Read the model definition and answer for the solid it produces. Units are mm, in the model's axes. A direction names the side the tool comes from. Round coordinates to 2 decimals unless told otherwise and drop trailing zeros. Write each loop counter-clockwise with the first axis right and the second up, starting at its lowest first coordinate (ties: lowest second). Pieces come first, ordered by that corner, then holes.
from build123d import *

# Parameters (mm, degrees)
F1_DEPTH = 65.0748
F3_DEPTH = 69.851
F4_R     = 17.4498
F5_DEPTH = 25.4
F6_R     = 6.35
F7_DEPTH = 30.1498
F8_R     = 3.175
F9_DEPTH = 15.875
F10_F1_R = 3.175
F10_F2_R = 3.175


with BuildPart() as f1:
    # F0 (on Right) → F1 (new body)
    with BuildSketch(Plane.YZ):
        Polygon((32.8030504316, 53.1119473694), (-37.0469495684, 53.1119473694), (-37.0469495684, 8.6619473694), (-14.8219495684, 8.6619473694), (-14.8219495684, -4.1650526306), (-9.2339495684, -4.1650526306), (-9.2339495684, -8.9275526306), (-14.8219495684, -8.9275526306), (-14.8219495684, -29.4380526306), (10.5780504316, -29.4380526306), (10.5780504316, -8.9275526306), (4.9900504316, -8.9275526306), (4.9900504316, -4.1650526306), (10.5780504316, -4.1650526306), (10.5780504316, 8.6619473694), (32.8030504316, 8.6619473694), align=None)
    extrude(amount=F1_DEPTH)

    # F2 (on face) → F3 (cut, through all)
    with BuildSketch(Plane.XZ.offset(37.0469495684)):
        with BuildLine():
            ThreePointArc((22.225, 5.4869473694), (24.4700640303, 6.4168833391), (25.4, 8.6619473694))
            Line((25.4, 8.6619473694), (0, 8.6619473694))
            Line((0, 8.6619473694), (0, -29.4380526306))
            Line((0, -29.4380526306), (9.525, 5.4869473694))
            Line((9.525, 5.4869473694), (22.225, 5.4869473694))
        make_face()
        Polygon((25.4, 27.7119473694), (25.4, 53.1119473694), (0, 53.1119473694), (0, 8.6619473694), (25.4, 8.6619473694), align=None)
        with BuildLine():
            Line((65.0748, 53.1119473694), (39.8529659904, 53.1119473694))
            ThreePointArc((39.8529659904, 53.1119473694), (51.2636522621, 42.3660722249), (56.8255061373, 27.7119473694))
            Line((56.8255061373, 27.7119473694), (65.0748, 27.7119473694))
            Line((65.0748, 27.7119473694), (65.0748, 53.1119473694))
        make_face()
    extrude(amount=-F3_DEPTH, mode=Mode.SUBTRACT)

    # F4 (on face) → F5 (join)
    with BuildSketch(Plane.YZ.offset(65.0748)):
        with Locations((-2.1219495684, 26.1117473694)):
            Circle(F4_R)
    extrude(amount=-F5_DEPTH)

    # F6 (on face) → F7 (cut)
    with BuildSketch(Plane.YZ.offset(65.0748)):
        with Locations((-2.1219495684, 26.1117473694)):
            Circle(F6_R)
    extrude(amount=-F7_DEPTH, mode=Mode.SUBTRACT)

    # F8 (on face) → F9 (cut)
    with BuildSketch(Plane(origin=(25.4, 0, 0), x_dir=(0, -1, 0), z_dir=(-1, 0, 0))):
        with Locations((-16.9280504316, 34.0619473694)):
            Circle(F8_R)
        with Locations((21.1719495684, 34.0619473694)):
            Circle(F8_R)
    extrude(amount=-F9_DEPTH, mode=Mode.SUBTRACT)

    # F10: fillet of radius 3.175 on 12 edges, made by hand

    # F10_f1
    f10_f1_edges = [f1.edges().sort_by_distance(p)[0] for p in [
        (50.428197841, -2.1264417395, 43.5615467912),
        (56.8255061373, -28.2725863076, 27.7119473694),
        (56.8255061373, 24.0286871709, 27.7119473694),
    ]]
    fillet(f10_f1_edges, radius=F10_F1_R)

    # F10_f2
    f10_f2_edges = [f1.edges().sort_by_distance(p)[0] for p in [
        (50.5351306509, -37.0469495684, 43.4143386342),
        (62.2832541328, -37.0469495684, 27.7119473694),
        (65.0748, 32.8030504316, 18.1869473694),
        (50.5351306509, 32.8030504316, 43.4143386342),
        (39.8529659904, -2.1219495684, 53.1119473694),
        (65.0748, -28.2725863076, 27.7119473694),
        (65.0748, -2.1219495684, 43.5615473694),
        (65.0748, 24.0286871709, 27.7119473694),
        (65.0748, -37.0469495684, 18.1869473694),
        (57.4937274099, 32.8030504316, 28.4194187475),
        (57.4937274099, -37.0469495684, 28.4194187475),
    ]]
    fillet(f10_f2_edges, radius=F10_F2_R)


solid = f1.part
Q1. Which of the six approach directions +Z, -Z, +X, -X, +Y, -Y give full straight-line access (tool end or side, diameter ignored) to faces 1 (the cylindrical face through (48.77, -2.57, 45.66)), 2 (the cylindrical face through (64.169, -26.919, 26.757)), 3 (the flat face through (45, 22, 8.662))?
Verdict:
face 1: +Z, +X
face 2: +Z, +X, -Y
face 3: -Z, +X, -X, +Y
Q2. Determine the mould class of faces 4 (the flat face through (16, -2, 5.487)), 5 (the flat face through (39, -37.047, 26)), 6 (the cylindrical face through (33.226, -22.637, 31.245)) for opening direction Z: pulls with the +Z half, pulls with the -Z half, needs draft (parallel to the pull), parting line crosses it, or undercut.
Verdict:
face 4: pulls with the +Z half
face 5: needs draft
face 6: undercut
Q3. Section A-A (x = 21) is taken. Determine the outline of the cut face in (y, z), then the cut area to 3 significant figures.
Verdict:
outline: (-14.82, -29.44) - (10.58, -29.44) - (10.58, -8.93) - (4.99, -8.93) - (4.99, -4.17) - (10.58, -4.17) - (10.58, 5.49) - (-14.82, 5.49) - (-14.82, -4.17) - (-9.23, -4.17) - (-9.23, -8.93) - (-14.82, -8.93) - close
area: 834 mm2
Q4. Section D-D (x = 8.5) is taken. Determine the outline of the cut face in (y, z), then the cut area to 3 significant figures.
Verdict:
outline: (-14.82, -29.44) - (10.58, -29.44) - (10.58, -8.93) - (4.99, -8.93) - (4.99, -4.17) - (10.58, -4.17) - (10.58, 1.73) - (-14.82, 1.73) - (-14.82, -4.17) - (-9.23, -4.17) - (-9.23, -8.93) - (-14.82, -8.93) - close
area: 738 mm2
Q5. Section B-B (y = -27.5) is taken. Determine the outline of the cut face in (x, z) (3 decimals), then the cut area to 3 significant figures.
Verdict:
outline: (25.4, 8.662) - (65.075, 8.662) - (65.075, 24.537) arc R3.175 ccw to (61.9, 27.712) - (59.492, 27.712) arc R3.175 cw to (56.386, 30.227) arc R34.925 ccw to (40.645, 52.634) arc R3.175 ccw to (38.971, 53.112) - (25.4, 53.112) - close
area: 1,410 mm2
Q6. Section C-C (z = 16) is taken. Determine the outline of the cut face in (x, y) (3 decimals).
Verdict:
outline: (25.4, -37.047) - (61.9, -37.047) arc R3.175 ccw to (65.075, -33.872) - (65.075, 29.628) arc R3.175 ccw to (61.9, 32.803) - (25.4, 32.803) - close
Q7. Straight lines are drawn through the part: probe 1 along Z at (x, y) = (31, -11); probe 2 along X at (y, z) = (-7, 23) (3 decimals); probe 3 along Y at (x, z) = (35, 0). For each, find the intervals that lie inside material, in ascending order.
Verdict:
probe 1: z = -29.44 to -8.93, -4.17 to 53.11
probe 2: x = 25.4 to 34.925
probe 3: y = -14.82 to 10.58
Q8. Flat-ended cylindrical pins translate along their axes: pin 1 Ø2 at (x, y) = (53, -21) entering from -Z; pin 2 Ø10 at (y, z) = (-21.17, 34.06) entering from -X; pin 3 Ø11.5 at (y, z) = (-2.12, 26.11) entering from +X (3 decimals). Find the tip coordinate at first contact, or state that the pin passes through.
Verdict:
pin 1: stops at z = 8.66
pin 2: stops at x = 25.4
pin 3: stops at x = 34.925
